CAD build for the part. Positions are in the model's coordinates, mm. A direction names the side the tool comes from. Give positions to 0.01 mm unless a question says otherwise; leave off trailing zeros. Order: outer loops, then holes, each group sorted by start corner. A loop starts at its lowest first (then second) coordinate and runs counter-clockwise, first axis right, second up. Notation, with made-up numbers: (13.5, 77.25) -> (55.5, 77.25) arc R16 ccw to (55.5, 88.25) -> close; hole circle Ø8 at (-20, -26). An arc over 180 degrees is marked (long way). Use one line per item in the form item = value. Start each with the question number.
1) Cut at D-D, the plane z = 0. Give the cut face in (x, y), and give its area (3 significant figures).
2) Mould opens along Z. For faces 1 (the face through (6.5, 0, 6)), 2 (the face through (3, -1.95, -1)), 3 (the face through (3.451, -0.748, -0.976)) say: pulls with the +Z half, pulls with the -Z half, needs draft (parallel to the pull), parting line crosses it, or undercut.
3) Cut at B-B, the plane y = 0. Give the cut face in (x, z), and give its area (3 significant figures).
4) Cut at A-A, the plane z = 5. Give the cut face in (x, y), and give its area (3 significant figures).
5) Probe line 1 (Z direction, x = 4.5, y = 0); line 2 (Y direction, x = 4, z = 0); line 3 (X direction, y = 1, z = 5.25). List the from-to ranges inside material, lowest first.
6) Tool access for faces 4 (the face through (6, 0, 4)), 5 (the face through (7, 0, -1.4)): list every direction of +Z, -Z, +X, -X, +Y, -Y with a clear straight run to the whole face (end or side of a thin tool).
7) Cut at C-C, the plane x = 0.5. Give the cut face in (y, z), and give its area (3 significant figures).
8) Drop flat-ended pins along their axis: P1, Ø1.1, axis at y = 0.5, z = 4, coming from the -X side; P2, Ø1.5, axis at x = 4, y = -1, coming from the +Z side. Give the stop position or say it passes through.
Solid Edge part; units mm, degrees
sketch "Sketch1" plane through (0, 0, 0) normal (1, 0, 0) x (0, 1, 0)
  line L0 (-1.95, -6) -> (1.95, -6)
  line L1 (1.95, -6) -> (1.95, 6)
  line L2 (1.95, 6) -> (-1.95, 6)
  line L3 (-1.95, 6) -> (-1.95, -6)
  dimension "D1" = 1.95
  dimension "D2" = 1.95
extrude "Protrusion1" add sketch "Sketch1" along normal blind 7
hole "Bohrung_2" at (0, 0, 0) direction (1, 0, 0) diameter 2.459 end up to next
sketch "Sketch2" plane through (3.5, -1.95, 0) normal (0, -1, 0) x (1, 0, 0)
  line L0 (-2.5, 6) -> (-2.5, 2)
  line L1 (-2.5, 2) -> (2.5, 2)
  line L2 (2.5, 2) -> (2.5, 6)
  dimension "D1" = 2.5
  dimension "D2" = 2.5
extrude "Extrusionsausschnitt_2" cut sketch "Sketch2" along normal mid plane 9.7632 material side at (1.05, -1.95, 4)
fillet "Verrundung_2" radius 0.2 2 edges at (1, 0, 2) (6, 0, 2)
properties part number "052" material "Aluminiumlegierung:3.0205, Al 99.0, EN-AW 1200"
Result:
q1.outline = (0, -1.95) -> (7, -1.95) -> (7, -1.23) -> (0, -1.23) -> close; (0, 1.23) -> (7, 1.23) -> (7, 1.95) -> (0, 1.95) -> close
q1.area = 10.1 mm²
q2.face_1 = pulls with the +Z half
q2.face_2 = needs draft
q2.face_3 = undercut
q3.outline = (0, -6) -> (7, -6) -> (7, -1.23) -> (0, -1.23) -> close; (0, 1.23) -> (7, 1.23) -> (7, 6) -> (6, 6) -> (6, 2.2) arc R0.2 cw to (5.8, 2) -> (1.2, 2) arc R0.2 cw to (1, 2.2) -> (1, 6) -> (0, 6) -> close
q3.area = 46.8 mm²
q4.outline = (0, -1.95) -> (1, -1.95) -> (1, 1.95) -> (0, 1.95) -> close; (6, -1.95) -> (7, -1.95) -> (7, 1.95) -> (6, 1.95) -> close
q4.area = 7.80 mm²
q5.line_1 = -6 to -1.23, 1.23 to 2
q5.line_2 = -1.95 to -1.23, 1.23 to 1.95
q5.line_3 = 0 to 1, 6 to 7
q6.face_4 = +Z, +Y, -Y
q6.face_5 = +Z, -Z, +X, +Y, -Y
q7.outline = (-1.95, -6) -> (1.95, -6) -> (1.95, 6) -> (-1.95, 6) -> close; hole circle Ø2.46 at (0, 0)
q7.area = 42.1 mm²
q8.P1 = 0
q8.P2 = 2
